Source: three-view drawing plus pictorial views. Frame: mm from the lowest corner of the part. Give positions to 0.01 mm unless a question says otherwise; leave off trailing zeros. Loops run counter-clockwise (first coordinate to the right, second up) from the corner with the lowest first, then second, coordinate; pieces in that order, holes last. Notation, with made-up numbers: (60.25, -39.5) -> (84.25, -39.5) arc R18 cw to (84.25, -8.5) -> close; hole circle Ø7 at (-34.5, -32.75). An arc over 180 degrees is marked (long way). Put each result on its own line as item: value.
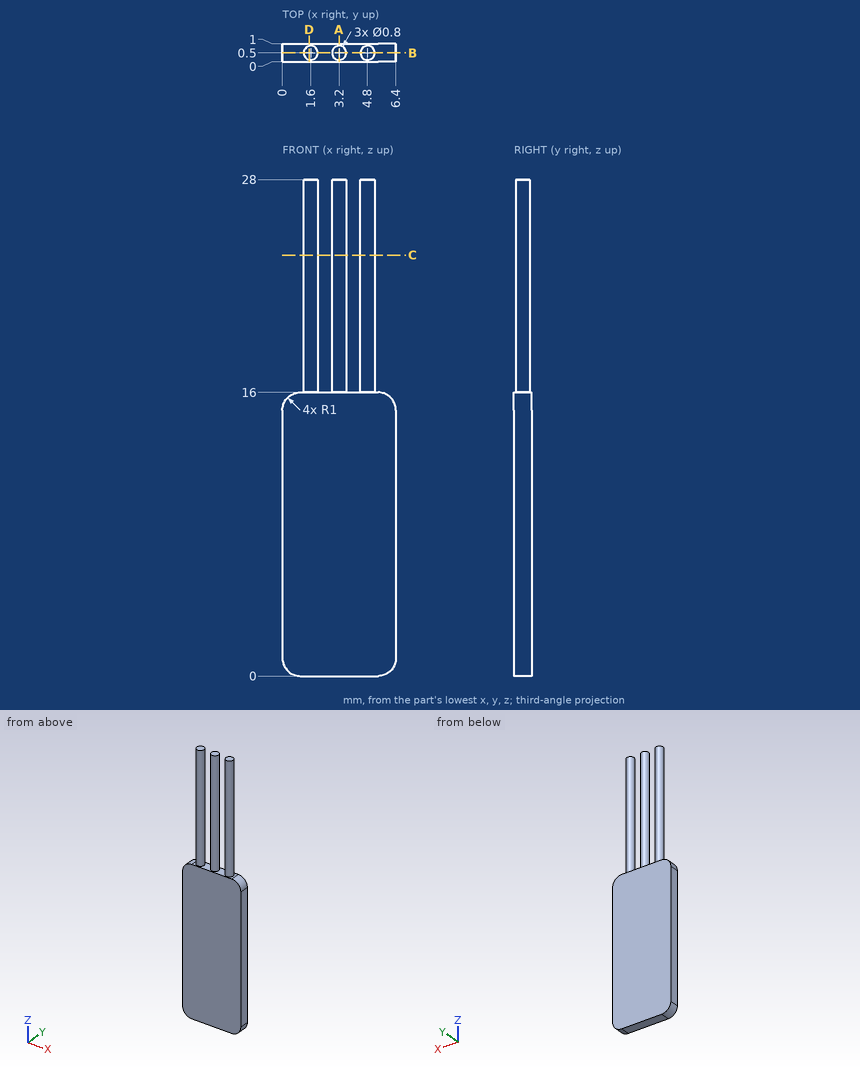
(1) Section B-B on y = 0.5. Return loops of the section in (x, z).
Calculated:
outline: (0, 1) arc R1 ccw to (1, 0) -> (5.4, 0) arc R1 ccw to (6.4, 1) -> (6.4, 15) arc R1 ccw to (5.4, 16) -> (5.2, 16) -> (5.2, 28) -> (4.4, 28) -> (4.4, 16) -> (3.6, 16) -> (3.6, 28) -> (2.8, 28) -> (2.8, 16) -> (2, 16) -> (2, 28) -> (1.2, 28) -> (1.2, 16) -> (1, 16) arc R1 ccw to (0, 15) -> close
(2) Section D-D on x = 1.5. Return loops of the section in (y, z), then the cut area to 3 significant figures.
Calculated:
outline: (0, 0) -> (1, 0) -> (1, 16) -> (0.89, 16) -> (0.89, 28) -> (0.11, 28) -> (0.11, 16) -> (0, 16) -> close
area: 25.3 mm²
(3) Section A-A on x = 3.2. Return loops of the section in (y, z), then the cut area to 3 significant figures.
Calculated:
outline: (0, 0) -> (1, 0) -> (1, 16) -> (0.9, 16) -> (0.9, 28) -> (0.1, 28) -> (0.1, 16) -> (0, 16) -> close
area: 25.6 mm²
(4) First-contact query: P1, Ø1, axis at x = 5, z = 7.5, coming from the -Y side. Flat tip, straight axial feed; report the tip coordinate or a pass-through.
Calculated:
P1: stops at y = 0
(5) Line query: probe 1 along X at (y, z) = (0.3, 25); probe 2 along Y at (x, z) = (3.25, 16.5); probe 3 along Z at (x, y) = (5.5, 0.2). Output: solid intervals per line, ascending. Write a range as from..to.
Calculated:
probe 1: x = 1.25..1.95, 2.85..3.55, 4.45..5.15
probe 2: y = 0.1..0.9
probe 3: z = 0.01..15.99
(6) Section C-C on z = 23.75. Return loops of the section in (x, y).
Calculated:
outline: circle Ø0.8 at (1.6, 0.5); circle Ø0.8 at (3.2, 0.5); circle Ø0.8 at (4.8, 0.5)
